Read the model definition and answer for the solid it produces. Units are mm, in the model's axes. Face numbers are marked on the shaded views. A direction names the side the tool comes from. Coordinates: 2 decimals unless noted, no trailing zeros. Write each loop counter-clockwise with the first axis right and the second up, starting at its lowest first coordinate (ties: lowest second). Pieces come first, ordered by that corner, then holes. Notation, with made-up numbers: (49.5, -9) -> (99.5, -9) arc R24 cw to (99.5, 25) -> close; hole circle Ø6 at (13.5, 22.25). An arc over 180 degrees is marked (long way). Answer as a JSON object with one key per item and string values. Group by question number.
(1) Flat-ended cylindrical pins translate along their axes: P1, Ø6.5, axis at x = -18.5, z = 5, coming from the +Y side; P2, Ø1.5, axis at y = 16.5, z = 8, coming from the -X side; P3, Ø5, axis at x = -9, z = 10, coming from the -Y side. Find the tip coordinate at first contact, or state that the pin passes through.
(2) Straight lines are drawn through the part: L1, parallel to X at y = -5, z = 8.5; L2, parallel to X at y = -9.5, z = 6.75; L3, parallel to Y at x = -11.75, z = 2.5. For each, find the intervals that lie inside material, in ascending order.
(3) Which of the six approach directions +Z, -Z, +X, -X, +Y, -Y give full straight-line access (tool end or side, diameter ignored) to the marked faces 1, 2, 3, 4 and 5?
(4) Find section A-A (z = 2). Give the vertices of the cut face in (x, y).
(5) Find section B-B (y = -2). Give the vertices of the cut face in (x, z).
(6) Find section C-C (x = -8.5). Give the vertices of the cut face in (y, z).
from build123d import *

# Parameters (mm, degrees)
F0_W     = 4.2672
F0_H     = 14.351
F0_W_2   = 2.286
F0_H_2   = 5.1308
F0_W_3   = 2.154207
F0_H_3   = 5.1562
F1_DEPTH = 12.2936


with BuildPart() as f1:
    # F0 (on Top) → F1 (new body)
    with BuildSketch(Plane.XY):
        Polygon((-13.986457, 14.351), (-17.999657, 14.351), (-17.999657, 0), (-17.999657, -7.6454), (-13.986457, -7.6454), (-11.83225, -7.6454), (4.504743, -7.6454), (4.504743, 14.351), (-11.700457, 14.351), align=None)
        with Locations((-20.133257, 7.1755)):
            Rectangle(F0_W, F0_H)
        with Locations((-12.843457, 16.9164)):
            Rectangle(F0_W_2, F0_H_2)
        with Locations((-12.909353, -10.2235)):
            Rectangle(F0_W_3, F0_H_3)
    extrude(amount=F1_DEPTH)


solid = f1.part
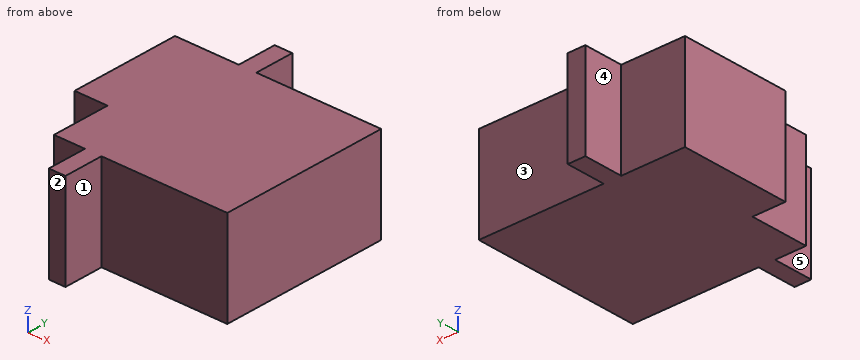
Results below:
{
 "1": {"P1": "stops at y = 14.35", "P2": "stops at x = -13.99", "P3": "stops at y = -7.65"},
 "2": {"L1": "x = -18 to 4.5", "L2": "x = -13.99 to -11.83", "L3": "y = -7.65 to 19.48"},
 "3": {"face 1": "+Z, -Z, +X, -Y", "face 2": "+Z, -Z, +X, -X, -Y", "face 3": "+Z, -Z, +X, +Y", "face 4": "+Z, -Z, -X, +Y", "face 5": "+Z, -Z, -X, -Y"},
 "4": {"outline": "(-22.27, 0) -> (-18, 0) -> (-18, -7.65) -> (-13.99, -7.65) -> (-13.99, -12.8) -> (-11.83, -12.8) -> (-11.83, -7.65) -> (4.5, -7.65) -> (4.5, 14.35) -> (-11.7, 14.35) -> (-11.7, 19.48) -> (-13.99, 19.48) -> (-13.99, 14.35) -> (-22.27, 14.35) -> close"},
 "5": {"outline": "(-18, 0) -> (4.5, 0) -> (4.5, 12.29) -> (-18, 12.29) -> close"},
 "6": {"outline": "(-7.65, 0) -> (14.35, 0) -> (14.35, 12.29) -> (-7.65, 12.29) -> close"}
}
